Check sheet for the modelled part. Datum: model origin and axes. Units: mm. A direction names the side the tool comes from. Give positions to 0.01 mm unless a question says otherwise; leave off trailing zeros. Write each question's results on one line, items separated by ' | '. Start each with the question number.
Item 1: Cross-section at A-A on y = 4.5. State how many separate pieces and enclosed holes the cut face has, then the cut area to 3 significant figures.
Item 2: Access from +Z, -Z, +X, -X, +Y, -Y to the whole of each face (thin tool, end or side, straight path). Record for faces 4 (the face through (0, 5.5, 0)), 5 (the face through (0, 15, 0)).
Item 3: Gauge pin test, flat ends, axial feed: pin 1 Ø1.5 at (y, z) = (8.5, -4.5) entering from +X; pin 2 Ø1 at (y, z) = (9.5, 7) entering from -X; pin 3 Ø1.5 at (x, z) = (8, 2.5) entering from -Y; pin 4 Ø1.7 at (x, y) = (0.5, 3.5) entering from -Z. Record the tip position at first contact, or that the pin passes through.
Item 4: Mould release check, pull along Z, two halves, no side actions. Record for faces 1 (the face through (-0.829, 7.395, 12.472)), 2 (the face through (-14.985, 7.395, 0.66)), 3 (the face through (3, 0, 0)): pulls with the +Z half, pulls with the -Z half, needs draft (parallel to the pull), parting line crosses it, or undercut.
Item 5: Scan lines: line 1 along X through (y, z) = (8.75, 3.5); line 2 along X through (y, z) = (10, -8.5); line 3 along Z through (x, y) = (4, 12.5). Record each from-to range of solid material in increasing order.
from build123d import *

# Parameters (mm, degrees)
F0_R            = 15
F1_DEPTH        = 15
F3_DEPTH        = 5.5
F5_DEPTH        = 15.001
F5_COPIES_COUNT = 6


# Not quite as in the source:
# - a pattern or mirror of a feature is missing from the dataset's text; its kind, count and spacing are read off the source's solid


with BuildPart() as f1:
    # F0 (on Front) → F1 (new body)
    with BuildSketch(Plane.XZ):
        Circle(F0_R)
    extrude(amount=-F1_DEPTH)

    # F2 (on face) → F3 (cut)
    with BuildSketch(Plane.XZ):
        with BuildLine():
            ThreePointArc((-1.0499999991, 1.000000001), (-0.5385164813, -1.3462912015), (1.45, 0))
            ThreePointArc((1.45, 0), (1.3462912015, 0.5385164813), (1.0499999991, 1.000000001))
            Line((1.0499999991, 1.000000001), (-1.0499999991, 1.000000001))
        make_face()
    extrude(amount=-F3_DEPTH, mode=Mode.SUBTRACT)

    # F4 (on face) → F5 (cut, through all)
    with BuildSketch(Plane.XZ):
        with BuildLine():
            ThreePointArc((2.6320639833, 12.2197479183), (-0.8786691083, 12.4690793805), (-4.3197418021, 11.7298691708))
            add(Edge.make_bspline(
                [(-4.3197418021, 11.7298691708), (-1.5711041633, 9.9351070821), (0, 6.4156376757), (0, 2.5)],
                knots=[0, 0, 0, 0, 10.1907141136, 10.1907141136, 10.1907141136, 10.1907141136], degree=3))
            ThreePointArc((0, 2.5), (0.3749457354, 2.4717232239), (0.7414096655, 2.3875325564))
            add(Edge.make_bspline(
                [(2.6320639833, 12.2197479183), (3.8345751818, 8.3321332932), (2.9968102463, 6.907931529), (0.7414096655, 2.3875325564)],
                knots=[0, 0, 0, 0, 10.0123440149, 10.0123440149, 10.0123440149, 10.0123440149], degree=3))
        make_face()
    f5 = extrude(amount=-F5_DEPTH, mode=Mode.SUBTRACT)

    # F5_copies: F5 ×6 about axis
    f5_copies_axis = Axis((0, 0, 0), (0, 1, 0))
    for i in range(1, F5_COPIES_COUNT):
        add(f5.rotate(f5_copies_axis, i * 360 / F5_COPIES_COUNT), mode=Mode.SUBTRACT)


solid = f1.part
Answer sheet:
1) separate pieces: 1 | enclosed holes: 7 | area: 472 mm²
2) face 4: -Y | face 5: +Z, -Z, +X, -X, +Y
3) pin 1: stops at x = 14.52 | pin 2: stops at x = -13.52 | pin 3: passes through | pin 4: stops at z = -15
4) face 1: undercut | face 2: parting line crosses it | face 3: needs draft
5) line 1: x = -14.59 to -12, -2.8 to -0.03, 1.3 to 5.09, 11.59 to 14.59 | line 2: x = -12.36 to -9.17, -7.86 to -3.15, 1.42 to 12.36 | line 3: z = -14.46 to -11.84, -11.51 to -5.19, -2.14 to 0.65, 2.51 to 14.46
